Read the model definition and answer for the solid it produces. Units are mm, in the model's axes. A direction names the side the tool comes from. Give positions to 0.01 mm unless a question says otherwise; leave off trailing zeros. Loops run counter-clockwise (first coordinate to the right, second up) from the corner with the lowest first, then second, coordinate; pieces in that order, holes last. Notation, with made-up numbers: (-33.5, 81.5) -> (17.5, 81.5) arc R15 ccw to (17.5, 107.5) -> close; hole circle Ø6 at (-28.5, -18.5). An arc over 180 degrees is marked (long way). Write each question's results on one line, items separated by ' | '. Start each with the question number.
Item 1: Section B-B on z = 10 is taken. Write down the section's boundary in (x, y).
Item 2: Section C-C on x = 12 is taken. Write down the section's boundary in (y, z).
Item 3: Which of the six approach directions +Z, -Z, +X, -X, +Y, -Y give full straight-line access (tool end or side, diameter ignored) to faces 1 (the flat face through (0, -7, -12)), 2 (the flat face through (-2, 10, -12)), 3 (the flat face through (-2, 6, 0)), 4 (the flat face through (-2, -7, 0))?
Item 4: Each of these flat-tipped pins is pushed along its axis until it touches: P1, Ø2.5, axis at x = -1.5, z = 7, coming from the +Y side; P2, Ø16.5, axis at y = -4, z = -15.5, coming from the +X side; P3, Ø10, axis at y = -2.5, z = -7.5, coming from the +X side. Where does it stop, or does it pass through?
Item 5: Find the intervals of material crossed by line 1 (X direction, y = -9, z = -13); line 2 (Y direction, x = 12.75, z = 8.5); line 3 (Y direction, x = -2, z = -15.5), in increasing order.
Item 6: Section D-D on y = -4 is taken. Write down the section's boundary in (x, z) (3 decimals).
Item 7: Section A-A on y = 24.5 is taken. Write down the section's boundary in (x, z) (3 decimals).
Autodesk Fusion 360 part; units mm, degrees
sketch "Sketch1" plane through (0, 0, 0) normal (0, 1, 0) x (1, 0, 0)
  arc A0 (0, -23.375) -> (0, 23.375) centre (0, 0) ccw
  arc A1 (0, -23.375) -> (0, 23.375) centre (0, 0) ccw
  line L0 (0, -23.375) -> (0, 23.375)
extrude "Extrude1" add sketch "Sketch1" along normal blind 30
sketch "Sketch2" plane through (0, 0, 0) normal (-1, 0, 0) x (0, 0, 1)
  line L0 (-23.375, 0) -> (23.375, 0)
  line L1 (23.375, 0) -> (23.375, 30)
  line L2 (23.375, 30) -> (-23.375, 30)
  line L3 (-23.375, 30) -> (-23.375, 0)
  line L4 (-23.375, 10) -> (0, 10)
  line L5 (0, 10) -> (0, -15)
  line L6 (0, -15) -> (-23.375, -15)
  line L7 (-23.375, -15) -> (-23.375, 10)
extrude "Extrude2" add sketch "Sketch2" along normal blind 5 contours L0 L3 L4 L5 L7 | L0 L5 L6 L7
sketch "Sketch4" plane through (0, 0, 0) normal (0, 1, 0) x (1, 0, 0)
  line L0 (0, 0) -> (-5, 0)
  line L1 (-5, 0) -> (-5, -23.375)
  line L2 (-5, -23.375) -> (0, -23.375)
  line L3 (0, -23.375) -> (0, 0)
  point P0 (0, -23.375)
extrude "Extrude3" add sketch "Sketch4" along normal blind 1
Findings:
1) outline: (-5, 0) -> (21.13, 0) -> (21.13, 30) -> (0, 30) -> (0, 1) -> (-5, 1) -> close
2) outline: (0, -20.06) -> (30, -20.06) -> (30, 20.06) -> (0, 20.06) -> close
3) face 1: +Z, -Z, +X, -Y | face 2: +Z, -Z, -X, +Y | face 3: +Z, -X, +Y | face 4: +Z, +X, -X, -Y
4) P1: y = 1 | P2: x = 21.86 | P3: x = 23.16
5) line 1: -5 to 0 | line 2: 0 to 30 | line 3: -15 to 10
6) outline: (-5, -23.375) -> (0, -23.375) -> (0, 0) -> (-5, 0) -> close
7) outline: (0, -23.375) arc R23.375 ccw to (0, 23.375) -> close
